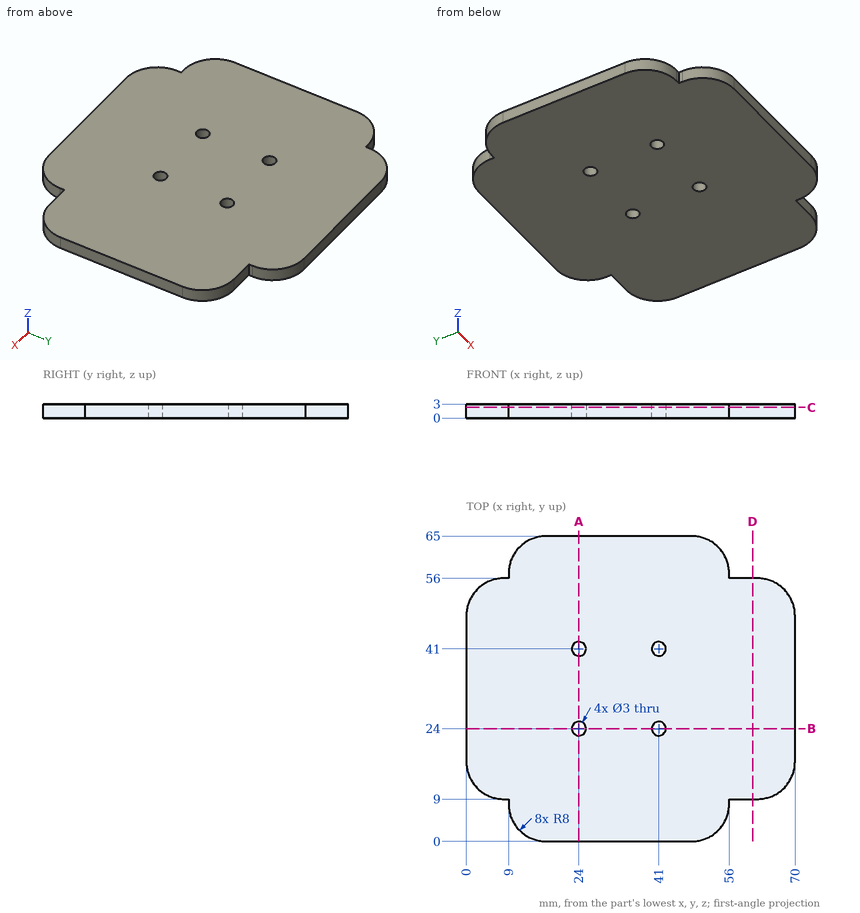
Source: three-view drawing plus pictorial views. Frame: mm from the lowest corner of the part. Round coordinates to 2 decimals unless told otherwise and drop trailing zeros. Loops run counter-clockwise (first coordinate to the right, second up) from the corner with the lowest first, then second, coordinate; pieces in that order, holes last. Notation, with made-up numbers: (18, 14) -> (57, 14) arc R16 cw to (57, 36) -> close; hole circle Ø6 at (13, -37). An arc over 180 degrees is marked (long way). Use one line per item in the form item = value.
Item 1: Cut plane A-A on x = 24. Output: boundary loops of the cut face in (y, z).
Evaluation:
outline = (0, 0) -> (22.5, 0) -> (22.5, 3) -> (0, 3) -> close; (25.5, 0) -> (39.5, 0) -> (39.5, 3) -> (25.5, 3) -> close; (42.5, 0) -> (65, 0) -> (65, 3) -> (42.5, 3) -> close
Item 2: Cut plane D-D on x = 61. Output: boundary loops of the cut face in (y, z), then the cut area to 3 significant figures.
Evaluation:
outline = (9, 0) -> (56, 0) -> (56, 3) -> (9, 3) -> close
area = 141 mm2
Item 3: Material intervals for probe 1 along Y at (x, z) = (41, 1.8); probe 2 along Y at (x, z) = (12.5, 2.7); probe 3 along Y at (x, z) = (64, 2.75), sorted ascending.
Evaluation:
probe_1 = 0 to 22.5, 25.5 to 39.5, 42.5 to 65
probe_2 = 1.39 to 63.61
probe_3 = 9.25 to 55.75
Item 4: Contact query for flat-ended pins moving along their axis: pin 1 Ø0.8 at (y, z) = (56.5, 1) entering from -X; pin 2 Ø0.5 at (y, z) = (56.5, 1) entering from +X; pin 3 Ø1 at (y, z) = (55, 2) entering from -X. Output: stop coordinate, or through.
Evaluation:
pin_1 = 9
pin_2 = 56
pin_3 = 3.34
Item 5: Cut plane B-B on y = 24. Output: boundary loops of the cut face in (x, z).
Evaluation:
outline = (0, 0) -> (22.5, 0) -> (22.5, 3) -> (0, 3) -> close; (25.5, 0) -> (39.5, 0) -> (39.5, 3) -> (25.5, 3) -> close; (42.5, 0) -> (70, 0) -> (70, 3) -> (42.5, 3) -> close
Item 6: Cut plane C-C on z = 2.3. Output: boundary loops of the cut face in (x, y).
Evaluation:
outline = (0, 17) arc R8 ccw to (8, 9) -> (9, 9) -> (9, 8) arc R8 ccw to (17, 0) -> (48, 0) arc R8 ccw to (56, 8) -> (56, 9) -> (62, 9) arc R8 ccw to (70, 17) -> (70, 48) arc R8 ccw to (62, 56) -> (56, 56) -> (56, 57) arc R8 ccw to (48, 65) -> (17, 65) arc R8 ccw to (9, 57) -> (9, 56) -> (8, 56) arc R8 ccw to (0, 48) -> close; hole circle Ø3 at (24, 24); hole circle Ø3 at (24, 41); hole circle Ø3 at (41, 24); hole circle Ø3 at (41, 41)
